Solid Edge part; units mm, degrees
sketch "Sketch1" plane through (0, 0, 0) normal (0, 0, 1) x (1, 0, 0)
  line L0 (25, -25) -> (25, 25)
  line L1 (25, 25) -> (-25, 25)
  line L2 (-25, 25) -> (-25, -25)
  line L3 (-25, -25) -> (25, -25)
extrude "Protrusion1" add sketch "Sketch1" along normal blind 93.2781
sketch "Sketch2" plane through (0, 0, 0) normal (1, 0, 0) x (0, 1, 0)
  line L0 (-25, 0) -> (0, 35.3553)
extrude "Cutout1" cut sketch "Sketch2" along normal up to next and the other way up to next material side at (0, -12.5408, 17.7065)
pattern_circular "Pattern1" count 4 over 360 about axis through (0, 0, 0) along (0, 0, 1) of "Cutout1"
mirror "Mirror1" about plane through (0, 0, 0) normal (0, 0, 1) of "Protrusion1", "Cutout1", "Pattern1"
Geometry: final body of the model. Coordinates: model frame, mm. Give positions to 0.01 mm unless a question says otherwise; leave off trailing zeros. Order: outer loops, then holes, each group sorted by start corner. A loop starts at its lowest first (then second) coordinate and runs counter-clockwise, first axis right, second up. Notation, with made-up numbers: (-38, -5) -> (-8, -5) arc R21 cw to (-8, 0) -> close; hole circle Ø8 at (-6, 80.5). An arc over 180 degrees is marked (long way). Answer as a JSON object with one key per item and string values.
Q1. Section D-D (z = 4.5). Output: boundary loops of the cut face in (x, y).
Entries:
{"outline": "(-21.82, -21.82) -> (21.82, -21.82) -> (21.82, 21.82) -> (-21.82, 21.82) -> close"}
Q2. Material intervals for probe 1 along Z at (x, y) = (-21.5, 4); probe 2 along Z at (x, y) = (-22, -19.5); probe 3 along Y at (x, z) = (21, 3.5), sorted ascending.
Entries:
{"probe 1": "z = -4.95 to 4.95", "probe 2": "z = -4.24 to 4.24", "probe 3": "y = -22.53 to 22.53"}
Q3. Section C-C (z = 24). Output: boundary loops of the cut face in (x, y), plus the area to 3 significant figures.
Entries:
{"outline": "(-8.03, -8.03) -> (8.03, -8.03) -> (8.03, 8.03) -> (-8.03, 8.03) -> close", "area": "258 mm^2"}
Q4. Section A-A (y = 21). Output: boundary loops of the cut face in (x, z).
Entries:
{"outline": "(-25, 0) -> (-21, -5.66) -> (21, -5.66) -> (25, 0) -> (21, 5.66) -> (-21, 5.66) -> close"}
Q5. First-contact query: pin 1 (5 mm diameter, centred on x = -6, y = -18, fed in from +Z) (3 decimals); pin 2 (1 mm diameter, centred on x = 10.5, y = 15.5, fed in from -Z); pin 3 (2 mm diameter, centred on x = 9, z = -7.5, fed in from +Y). Flat tips, straight axial feed; report the tip coordinate or a pass-through.
Entries:
{"pin 1": "stops at z = 13.435", "pin 2": "stops at z = -14.14", "pin 3": "stops at y = 20.4"}
Q6. Section B-B (x = 6). Output: boundary loops of the cut face in (y, z), plus the area to 3 significant figures.
Entries:
{"outline": "(-25, 0) -> (-6, -26.87) -> (6, -26.87) -> (25, 0) -> (6, 26.87) -> (-6, 26.87) -> close", "area": "1,670 mm^2"}
